Input: dimensioned drawing with shaded views. Units: mm. Origin: part minimum x, y, z. A direction names the side the tool comes from. Round coordinates to 2 decimals unless told otherwise and drop trailing zeros. Loops run counter-clockwise (first coordinate to the right, second up) from the corner with the lowest first, then second, coordinate; pieces in that order, holes last. Notation, with made-up numbers: M 12.5,30 L 35.5,30 A33 ccw 35.5,67 Z; hole C 52,54.5 d11. An arc over 180 degrees is marked long. One line per item, written item: value.
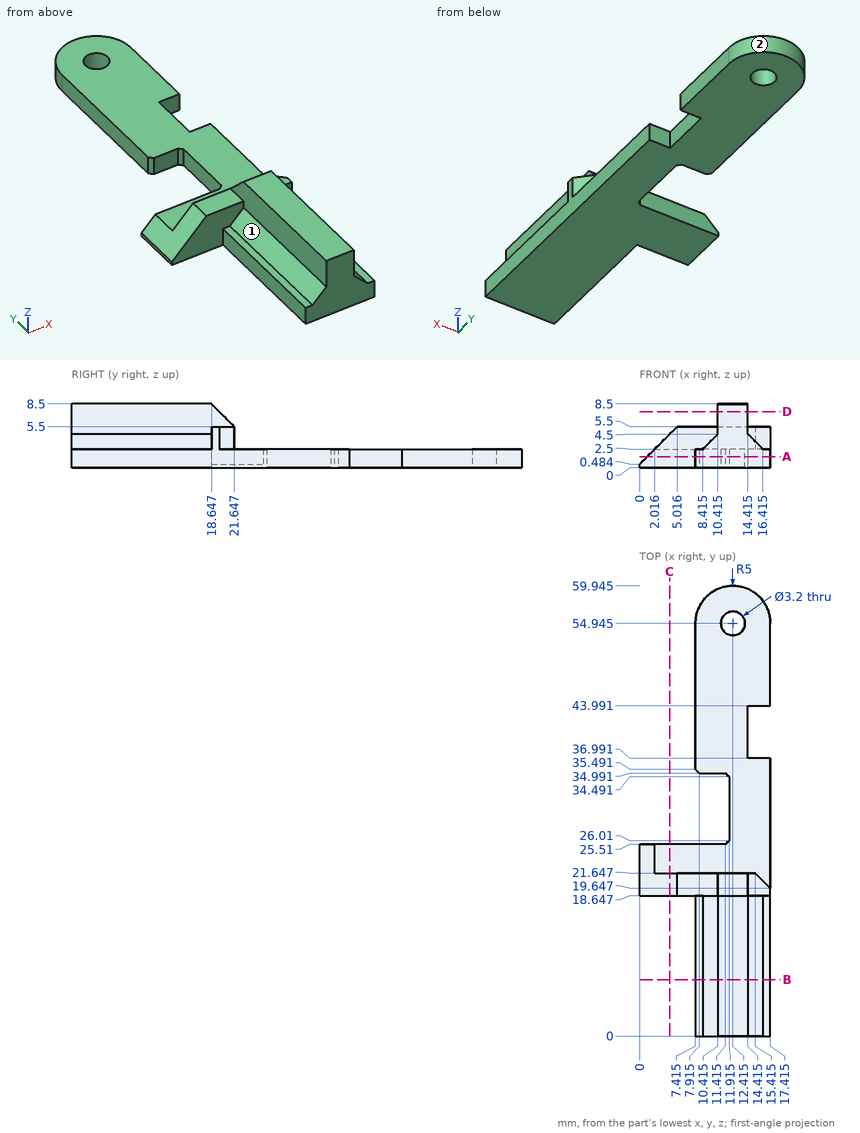
1. Pin query (flat end, axial travel): pin 1 (1.2 mm diameter, centred on y = 6, z = 6, fed in from -X) (3 decimals); pin 2 (4.5 mm diameter, centred on x = 10.5, y = 46, fed in from +Z); pin 3 (3 mm diameter, centred on x = 1.5, z = 3, fed in from -Y). Return the tip coordinate at first contact, or that it passes through.
Report:
pin 1: stops at x = 10.415
pin 2: stops at z = 2.5
pin 3: stops at y = 18.65
2. Ray query, line 1 (Y direction, x = 12, z = 3.5); line 2 (X direction, y = 29, z = 1) (1 decimal); line 3 (Y direction, x = 2.5, z = 2). Return the intervals inside material, ascending. Write a range as [from, to].
Report:
line 1: y = [0, 21.65]
line 2: x = [11.9, 17.4]
line 3: y = [18.65, 25.51]
3. Section query C-C (x = 4). Return the cut outline in (y, z) (1 decimal), and give its area (3 significant figures).
Report:
outline: M 18.6,0 L 25.5,0 L 25.5,2.5 L 21.6,2.5 L 21.6,4.5 L 18.6,4.5 Z
area: 23.1 mm2
4. Section query A-A (z = 1.5). Return the cut outline in (x, y) (1 decimal), and give its area (3 significant figures).
Report:
outline: M 1,18.6 L 7.4,18.6 L 7.4,0 L 17.4,0 L 17.4,37 L 14.4,37 L 14.4,44 L 17.4,44 L 17.4,54.9 A5 ccw 7.4,54.9 L 7.4,35.5 L 7.9,35 L 11.4,35 L 11.9,34.5 L 11.9,26 L 11.4,25.5 L 1,25.5 Z; hole C 12.4,54.9 d3.2
area: 561 mm2
5. Section query D-D (z = 7.5). Return the cut outline in (x, y) (1 decimal).
Report:
outline: M 10.4,0 L 14.4,0 L 14.4,19.6 L 10.4,19.6 Z
6. Section query B-B (y = 7.5). Return the cut outline in (x, z) (1 decimal).
Report:
outline: M 7.4,0 L 17.4,0 L 17.4,2.5 L 16.4,2.5 L 14.4,4.5 L 14.4,8.5 L 10.4,8.5 L 10.4,4.5 L 8.4,2.5 L 7.4,2.5 Z
7. Reachability of the marked faces 1 and 2 from +Z, -Z, +X, -X, +Y, -Y: full face, straight path, thin tool, end or side. Return the list, or none.
Report:
face 1: +Z, -X, -Y
face 2: +Z, -Z, +Y
